Autodesk Fusion 360 part; units mm, degrees
sketch "Sketch1" plane through (0, 0, 0) normal (0, 0, 1) x (1, 0, 0)
  line L0 (0, 0) -> (96, 0)
  line L1 (96, 0) -> (96, 46)
  line L2 (96, 46) -> (0, 46)
  line L3 (0, 46) -> (0, 0)
  dimension "d1" = 96
  dimension "d2" = 46
extrude "Extrude1" add sketch "Sketch1" along normal blind 2
fillet "Fillet1" radius 1 4 edges at (96, 0, 1) (96, 46, 1) (0, 0, 1) (0, 46, 1)
sketch "Sketch2" plane through (0, 0, 2) normal (0, 0, 1) x (-1, 0, 0)
  arc A0 (-1, -46) -> (0, -45) centre (-1, -45) ccw
  line L0 (0, -45) -> (0, -1)
  arc A1 (0, -1) -> (-1, 0) centre (-1, -1) ccw
  line L1 (-1, 0) -> (-95, 0)
  arc A2 (-95, 0) -> (-96, -1) centre (-95, -1) ccw
  line L2 (-96, -1) -> (-96, -45)
  arc A3 (-96, -45) -> (-95, -46) centre (-95, -45) ccw
  line L3 (-95, -46) -> (-1, -46)
  line L4 (-13.3, 0) -> (-26.73, 0)
  line L5 (-26.73, 0) -> (-26.73, -4.065)
  line L6 (-25.73, -5.065) -> (-14.3, -5.065)
  line L7 (-13.3, -4.065) -> (-13.3, 0)
  arc A4 (-14.3, -5.065) -> (-13.3, -4.065) centre (-14.3, -4.065) ccw
  arc A5 (-26.73, -4.065) -> (-25.73, -5.065) centre (-25.73, -4.065) ccw
  point P0 (-13.3, -5.065)
  dimension "d7" = 13.43
  dimension "d8" = 5.065
  dimension "d9" = 13.3
  dimension "d10" = 5.065
  dimension "d11" = 1
  dimension "d12" = 1
extrude "Extrude2" cut sketch "Sketch2" against normal blind 2 contours L1 L4 L5 L6 L7 A4 A5
fillet "Fillet4" radius 1 2 edges at (13.3, 0, 1) (26.73, 0, 1)
sketch "Sketch5" plane through (0, 0, 2) normal (0, 0, 1) x (-1, 0, 0)
  arc A0 (-26.73, -1) -> (-27.73, 0) centre (-27.73, -1) ccw
  line L0 (-27.73, 0) -> (-95, 0)
  arc A1 (-95, 0) -> (-96, -1) centre (-95, -1) ccw
  line L1 (-96, -1) -> (-96, -45)
  arc A2 (-96, -45) -> (-95, -46) centre (-95, -45) ccw
  line L2 (-95, -46) -> (-1, -46)
  arc A3 (-1, -46) -> (0, -45) centre (-1, -45) ccw
  line L3 (0, -45) -> (0, -1)
  arc A4 (0, -1) -> (-1, 0) centre (-1, -1) ccw
  line L4 (-1, 0) -> (-12.3, 0)
  arc A5 (-12.3, 0) -> (-13.3, -1) centre (-12.3, -1) ccw
  line L5 (-13.3, -1) -> (-13.3, -4.065)
  arc A6 (-14.3, -5.065) -> (-13.3, -4.065) centre (-14.3, -4.065) ccw
  line L6 (-14.3, -5.065) -> (-25.73, -5.065)
  arc A7 (-26.73, -4.065) -> (-25.73, -5.065) centre (-25.73, -4.065) ccw
  line L7 (-26.73, -4.065) -> (-26.73, -1)
  circle A8 centre (-5.1, -3.75) radius 1.6
  circle A9 centre (-5.1, -42.25) radius 1.6
  circle A10 centre (-90.9, -3.75) radius 1.6
  circle A11 centre (-90.9, -42.25) radius 1.6
  dimension "d33" = 3.2
  dimension "d34" = 3.75
  dimension "d35" = 5.1
  dimension "d36" = 3.2
  dimension "d37" = 3.75
  dimension "d38" = 5.1
  dimension "d39" = 3.2
  dimension "d40" = 5.1
  dimension "d41" = 3.75
  dimension "d42" = 3.2
  dimension "d43" = 3.75
  dimension "d44" = 5.1
extrude "Extrude5" cut sketch "Sketch5" against normal blind 2 contours A8 | A9 | A10 | A11
equation "d8 = 4.69 mm - 0.375 mm + 0.75 mm"
equation "d10 = 4.69 mm - 0.375 mm + 0.75 mm"
Source: CAD feature listing. Evaluate the final solid. Frame: model axes, mm. A direction names the side the tool comes from. Coordinates: 2 decimals unless noted, no trailing zeros. Order: outer loops, then holes, each group sorted by start corner. A loop starts at its lowest first (then second) coordinate and runs counter-clockwise, first axis right, second up. Notation, with made-up numbers: (15, 36.5) - (64, 36.5) arc R31 ccw to (64, 66.5) - close; hole circle Ø8 at (66, 80). An arc over 180 degrees is marked (long way). One line per item, written item: value.
1) Contact query for flat-ended pins moving along their axis: pin 1 (2.5 mm diameter, centred on x = 90.9, y = 3.75, fed in from -Z); pin 2 (1 mm diameter, centred on x = 21, z = 0.5, fed in from -Y) (3 decimals). Output: stop coordinate, or through.
Computed values:
pin 1: passes through
pin 2: stops at y = 5.065
2) Cut plane B-B on x = 90.9. Output: boundary loops of the cut face in (y, z), plus the area to 3 significant figures.
Computed values:
outline: (0, 0) - (2.15, 0) - (2.15, 2) - (0, 2) - close; (5.35, 0) - (40.65, 0) - (40.65, 2) - (5.35, 2) - close; (43.85, 0) - (46, 0) - (46, 2) - (43.85, 2) - close
area: 79.2 mm^2
3) Reachability of faces 4 (the face through (49, 46, 1)), 5 (the face through (13.3, 3, 1)) from +Z, -Z, +X, -X, +Y, -Y: full face, straight path, thin tool, end or side. Return the list, or none.
Computed values:
face 4: +Z, -Z, +X, -X, +Y
face 5: +Z, -Z, -Y
4) Cut plane A-A on y = 42.25. Output: boundary loops of the cut face in (x, z), plus the area to 3 significant figures.
Computed values:
outline: (0, 0) - (3.5, 0) - (3.5, 2) - (0, 2) - close; (6.7, 0) - (89.3, 0) - (89.3, 2) - (6.7, 2) - close; (92.5, 0) - (96, 0) - (96, 2) - (92.5, 2) - close
area: 179 mm^2
5) Ray query, line 1 (Y direction, x = 5.1, z = 0.95); line 2 (X direction, y = 42.25, z = 1.5); line 3 (X direction, y = 3.75, z = 1.55). Return the intervals inside material, ascending. Write a range as [from, to].
Computed values:
line 1: y = [0, 2.15], [5.35, 40.65], [43.85, 46]
line 2: x = [0, 3.5], [6.7, 89.3], [92.5, 96]
line 3: x = [0, 3.5], [6.7, 13.3], [26.73, 89.3], [92.5, 96]
6) Cut plane C-C on z = 0.6. Output: boundary loops of the cut face in (x, y) (3 decimals).
Computed values:
outline: (0, 1) arc R1 ccw to (1, 0) - (12.3, 0) arc R1 ccw to (13.3, 1) - (13.3, 4.065) arc R1 cw to (14.3, 5.065) - (25.73, 5.065) arc R1 cw to (26.73, 4.065) - (26.73, 1) arc R1 ccw to (27.73, 0) - (95, 0) arc R1 ccw to (96, 1) - (96, 45) arc R1 ccw to (95, 46) - (1, 46) arc R1 ccw to (0, 45) - close; hole circle Ø3.2 at (5.1, 3.75); hole circle Ø3.2 at (5.1, 42.25); hole circle Ø3.2 at (90.9, 3.75); hole circle Ø3.2 at (90.9, 42.25)
7) Mould query, pull axis Y, two halves, no side actions, for faces 1 (the face through (7, 0, 1)), 2 (the face through (89.374, 3.269, 1.014)), 3 (the face through (96, 23, 1)). Classes: released by +Y, released by -Y, zero draft, split by the parting line, or undercut.
Computed values:
face 1: released by -Y
face 2: undercut
face 3: zero draft
